from build123d import *

# Parameters (mm, degrees)
BOSS_EXTRUDE1_DEPTH     = 6.4
FILLET1_R               = 1
SKETCH2_R               = 0.5
BOSS_EXTRUDE2_DEPTH     = 0.2
SKETCH3_W               = 18.5
SKETCH3_H               = 0.1
SKETCH3_W_2             = 0.1
SKETCH3_H_2             = 1.2
BOSS_EXTRUDE3_DEPTH     = 6.4
BOSS_EXTRUDE4_DEPTH     = 6.4
SKETCH5_R               = 1.25
CUT_EXTRUDE1_DEPTH      = 29.157059506
SKETCH6_W               = 0.5
SKETCH6_H               = 4
BOSS_EXTRUDE5_DEPTH     = 6.4
FILLET2_R               = 0.2
CUT_EXTRUDE2_DEPTH      = 10
CUT_EXTRUDE3_DEPTH      = 25.523865927
CUT_EXTRUDE3_DEPTH_BACK = 25.523865927
SKETCH9_W               = 1
SKETCH9_H               = 1


with BuildPart() as part:
    # Sketch1 → Boss-Extrude1 (new body)
    with BuildSketch(Plane(origin=(0, 0, 0), x_dir=(1, 0, 0), z_dir=(0, 1, 0))):
        Polygon((0, 0), (20, 0), (20, 9.5), (10, 9.5), (9.3, 10.2), (0, 10.2), align=None)
    extrude(amount=BOSS_EXTRUDE1_DEPTH)

    # Fillet1
    fillet1_edges = [part.edges().sort_by_distance(p)[0] for p in [
        (0, 3.2, -10.2),
        (20, 3.2, -9.5),
        (20, 3.2, 0),
        (0, 3.2, 0),
    ]]
    fillet(fillet1_edges, radius=FILLET1_R)

    # Sketch2 → Boss-Extrude2 (add)
    with BuildSketch(Plane(origin=(0, 6.4, 0), x_dir=(1, 0, 0), z_dir=(0, 1, 0))):
        with Locations(Location((3.3, 9.2, 0), (0, 0, 90))):
            Circle(SKETCH2_R)
    extrude(amount=BOSS_EXTRUDE2_DEPTH)

    # Sketch3 → Boss-Extrude3 (add)
    with BuildSketch(Plane(origin=(0, 6.4, 0), x_dir=(1, 0, 0), z_dir=(0, 1, 0))):
        with BuildLine():
            ThreePointArc((3.3, 11.6), (3.370710678, 11.570710678), (3.4, 11.5))
            Line((3.4, 11.5), (21.9, 11.5))
            Line((21.9, 11.5), (21.9, 11.6))
            Line((21.9, 11.6), (3.3, 11.6))
        make_face()
        with Locations((12.65, 11.45)):
            Rectangle(SKETCH3_W, SKETCH3_H)
        with BuildLine():
            ThreePointArc((3.4, 11.5), (3.370710678, 11.429289322), (3.3, 11.4))
            Line((3.3, 11.4), (3.4, 11.4))
            Line((3.4, 11.4), (3.4, 11.5))
        make_face()
        with BuildLine():
            ThreePointArc((3.2, 11.5), (3.229289322, 11.429289322), (3.3, 11.4))
            Line((3.3, 11.4), (3.3, 11.5))
            Line((3.3, 11.5), (3.4, 11.5))
            ThreePointArc((3.4, 11.5), (3.370710678, 11.570710678), (3.3, 11.6))
            ThreePointArc((3.3, 11.6), (3.229289322, 11.570710678), (3.2, 11.5))
        make_face()
        with BuildLine():
            Line((3.3, 11.5), (3.3, 11.4))
            ThreePointArc((3.3, 11.4), (3.370710678, 11.429289322), (3.4, 11.5))
            Line((3.4, 11.5), (3.3, 11.5))
        make_face()
        with Locations((3.35, 10.8)):
            Rectangle(SKETCH3_W_2, SKETCH3_H_2)
        with BuildLine():
            Line((3.3, 10.2), (3.3, 11.4))
            ThreePointArc((3.3, 11.4), (3.229289322, 11.429289322), (3.2, 11.5))
            Line((3.2, 11.5), (3.2, 10.2))
            Line((3.2, 10.2), (3.3, 10.2))
        make_face()
    extrude(amount=-BOSS_EXTRUDE3_DEPTH)

    # Sketch4 → Boss-Extrude4 (add)
    with BuildSketch(Plane(origin=(0, 6.4, 0), x_dir=(1, 0, 0), z_dir=(0, 1, 0))):
        with BuildLine():
            Line((20.1, 11.6), (21.9, 11.6))
            Line((21.9, 11.6), (21.9, 14))
            ThreePointArc((21.9, 14), (21.4, 12.5), (20.1, 11.6))
        make_face()
        with BuildLine():
            ThreePointArc((18.7, 11.6), (19.046446609, 11.525126266), (19.4, 11.5))
            Line((19.4, 11.5), (19.4, 11.6))
            Line((19.4, 11.6), (18.7, 11.6))
        make_face()
        with BuildLine():
            Line((19.4, 11.6), (19.4, 11.5))
            ThreePointArc((19.4, 11.5), (19.753553391, 11.525126266), (20.1, 11.6))
            Line((20.1, 11.6), (19.4, 11.6))
        make_face()
        with BuildLine():
            Line((18.7, 11.6), (19.4, 11.6))
            Line((19.4, 11.6), (19.4, 16.5))
            ThreePointArc((19.4, 16.5), (17.632233047, 15.767766953), (16.9, 14))
            ThreePointArc((16.9, 14), (17.4, 12.5), (18.7, 11.6))
        make_face()
        with BuildLine():
            Line((19.4, 16.5), (19.4, 11.6))
            Line((19.4, 11.6), (20.1, 11.6))
            ThreePointArc((20.1, 11.6), (21.4, 12.5), (21.9, 14))
            ThreePointArc((21.9, 14), (21.167766953, 15.767766953), (19.4, 16.5))
        make_face()
        with BuildLine():
            Line((16.9, 11.6), (18.7, 11.6))
            ThreePointArc((18.7, 11.6), (17.4, 12.5), (16.9, 14))
            Line((16.9, 14), (16.9, 11.6))
        make_face()
    extrude(amount=-BOSS_EXTRUDE4_DEPTH)

    # Sketch5 → Cut-Extrude1 (cut, through all)
    with BuildSketch(Plane(origin=(0, 6.4, 0), x_dir=(1, 0, 0), z_dir=(0, 1, 0))):
        with Locations(Location((15, 2.5, 0), (0, 0, 270))):
            Circle(SKETCH5_R)
        with BuildLine():
            ThreePointArc((6.25, 2.5), (5, 3.75), (3.75, 2.5))
            Line((3.75, 2.5), (6.25, 2.5))
        make_face()
        with BuildLine():
            Line((6.25, 2.5), (3.75, 2.5))
            ThreePointArc((3.75, 2.5), (5, 1.25), (6.25, 2.5))
        make_face()
    extrude(amount=-CUT_EXTRUDE1_DEPTH, mode=Mode.SUBTRACT)

    # Sketch6 → Boss-Extrude5 (add)
    with BuildSketch(Plane(origin=(0, 6.4, 0), x_dir=(1, 0, 0), z_dir=(0, 1, 0))):
        with Locations((1.9, -2)):
            Rectangle(SKETCH6_W, SKETCH6_H)
        with Locations((10.7, -2)):
            Rectangle(SKETCH6_W, SKETCH6_H)
        with Locations((18, -2)):
            Rectangle(SKETCH6_W, SKETCH6_H)
    extrude(amount=-BOSS_EXTRUDE5_DEPTH)

    # Fillet2
    fillet2_edges = [part.edges().sort_by_distance(p)[0] for p in [
        (2.15, 3.2, 4),
        (1.65, 3.2, 4),
        (10.45, 3.2, 4),
        (10.95, 3.2, 4),
        (17.75, 3.2, 4),
        (18.25, 3.2, 4),
    ]]
    fillet(fillet2_edges, radius=FILLET2_R)

    # Sketch7 → Cut-Extrude2 (cut)
    with BuildSketch(Plane(origin=(0, 6.4, 0), x_dir=(1, 0, 0), z_dir=(0, 1, 0))):
        with BuildLine():
            ThreePointArc((18.7, 16.4), (19.046446609, 16.474873734), (19.4, 16.5))
            ThreePointArc((19.4, 16.5), (19.753553391, 16.474873734), (20.1, 16.4))
            Line((20.1, 16.4), (20.417508918, 16.4))
            Line((20.417508918, 16.4), (20.417508918, 16.594496766))
            Line((20.417508918, 16.594496766), (18.102606367, 16.594496766))
            Line((18.102606367, 16.594496766), (18.102606367, 16.4))
            Line((18.102606367, 16.4), (18.7, 16.4))
        make_face()
        with BuildLine():
            Line((19.4, 16.4), (19.4, 16.5))
            ThreePointArc((19.4, 16.5), (19.046446609, 16.474873734), (18.7, 16.4))
            Line((18.7, 16.4), (19.4, 16.4))
        make_face()
    extrude(amount=-CUT_EXTRUDE2_DEPTH, mode=Mode.SUBTRACT)

    # Sketch9 → Cut-Extrude3 (cut, two sides: drawn at the far end of the back side and taken through both)
    with BuildSketch(Plane.ZY.offset(-16.9).offset(-CUT_EXTRUDE3_DEPTH_BACK)):
        with Locations((-16, 3.7)):
            Rectangle(SKETCH9_W, SKETCH9_H)
        with Locations((-16, 2.7)):
            Rectangle(SKETCH9_W, SKETCH9_H)
    extrude(amount=CUT_EXTRUDE3_DEPTH + CUT_EXTRUDE3_DEPTH_BACK, mode=Mode.SUBTRACT)


solid = part.part
CAD build for the part. Positions are in the model's coordinates, mm. A direction names the side the tool comes from. Coordinates: 2 decimals unless noted, no trailing zeros. Loops run counter-clockwise (first coordinate to the right, second up) from the corner with the lowest first, then second, coordinate; pieces in that order, holes last. Notation, with made-up numbers: (45.5, 8) - (84.5, 8) arc R11 cw to (84.5, 24) - close; hole circle Ø7 at (71, 89.5). An arc over 180 degrees is marked (long way). Write item = value, one per line. Start each with the question number.
Q1. Flat gauge pins, fed straight in: pin 1 Ø1.5 at (x, z) = (19.5, 1.5) entering from -Y; pin 2 Ø1.1 at (y, z) = (4.5, 2) entering from -X; pin 3 Ø0.8 at (x, y) = (18.5, 2) entering from +Z; pin 4 Ø0.6 at (y, z) = (3, -11) entering from +X. Where does each tip first touch, or does it go through?
Q2. Cut at D-D, the plane z = -4.5. List the corners of the cut face in (x, y), then the cut area to 3 significant figures.
Q3. Pull direction Y, two halves, no side cores. Call faces 1 (the flat face through (0, 3, -5)), 2 (the flat face through (19, 2.2, -16)), 3 (the flat face through (11, 6.4, -6)): pulls with the +Y half, pulls with the -Y half, needs draft (parallel to the pull), parting line crosses it, or undercut.
Q4. Which spindle directions (+Z, -Z, +X, -X, +Y, -Y) get a long thin tool onto all of the face, cutting with end or side? Do faces 4 (the flat face through (3.4, 3, -11)), 5 (the flat face through (17.75, 3, 2)), 6 (the flat face through (3.2, 3, -11)), 7 (the flat face through (18.25, 3, 2)). Say none if no direction does.
Q5. Cut at C-C, the plane x = 15. List the corners of the cut face in (y, z).
Q6. Cut at A-A, the plane x = 5.75. List the corners of the cut face in (y, z).
Q7. Cut at B-B, the plane y = 4.75. Give the number of separate pieces and of enclosed holes in the cut face, then the cut area to 3 significant figures.
Q8. Drill centre lines: L1, parallel to Z at x = 5, y = 3.5; L2, parallel to Z at x = 13, y = 2.5; L3, parallel to Z at x = 4, y = 4. Where is each one in solid material? Low to high.
Computed:
q1.pin_1 = through
q1.pin_2 = 1.65
q1.pin_3 = 3.99
q1.pin_4 = 3.4
q2.outline = (0, 0) - (20, 0) - (20, 6.4) - (0, 6.4) - close
q2.area = 128 mm²
q3.face_1 = needs draft
q3.face_2 = undercut
q3.face_3 = pulls with the +Y half
q4.face_4 = +X, +Y, -Y
q4.face_5 = +Z, +Y, -Y
q4.face_6 = -Z, -X, +Y, -Y
q4.face_7 = +Z, +X, +Y, -Y
q5.outline = (0, -11.6) - (6.4, -11.6) - (6.4, -11.4) - (0, -11.4) - close; (0, -9.5) - (6.4, -9.5) - (6.4, -3.75) - (0, -3.75) - close; (0, -1.25) - (6.4, -1.25) - (6.4, 0) - (0, 0) - close
q6.outline = (0, -11.6) - (6.4, -11.6) - (6.4, -11.4) - (0, -11.4) - close; (0, -10.2) - (6.4, -10.2) - (6.4, -3.5) - (0, -3.5) - close; (0, -1.5) - (6.4, -1.5) - (6.4, 0) - (0, 0) - close
q7.separate_pieces = 1
q7.enclosed_holes = 2
q7.area = 218 mm²
q8.L1 = -11.6 to -11.4, -10.2 to -3.75, -1.25 to 0
q8.L2 = -11.6 to -11.4, -9.5 to 0
q8.L3 = -11.6 to -11.4, -10.2 to -3.25, -1.75 to 0
